```python
from build123d import *

# Parameters (mm, degrees)
SKETCH1_W           = 65
SKETCH1_H           = 46
SKETCH1_R           = 1.5
BOSS_EXTRUDE1_DEPTH = 5
SKETCH2_R           = 2
CUT_EXTRUDE1_DEPTH  = 10
SKETCH3_W           = 4
SKETCH3_H           = 46
CUT_EXTRUDE2_DEPTH  = 6
SKETCH4_W           = 6
SKETCH4_H           = 46
BOSS_EXTRUDE2_DEPTH = 5
FILLET1_R           = 10
FILLET2_R           = 1


with BuildPart() as part:
    # Sketch1 → Boss-Extrude1 (new body)
    with BuildSketch(Plane.XY):
        with Locations((7.5, 0)):
            Rectangle(SKETCH1_W, SKETCH1_H)
        with BuildLine():
            ThreePointArc((4.6, 0), (3.252691193, -3.252691193), (0, -4.6))
            ThreePointArc((0, -4.6), (-3.252691193, 3.252691193), (4.6, 0))
        make_face(mode=Mode.SUBTRACT)
        with Locations((30, -18.25)):
            Circle(SKETCH1_R, mode=Mode.SUBTRACT)
        with BuildLine():
            ThreePointArc((1.5, -10), (-1.060660172, -11.060660172), (0, -8.5))
            ThreePointArc((0, -8.5), (1.060660172, -8.939339828), (1.5, -10))
        make_face(mode=Mode.SUBTRACT)
        with BuildLine():
            ThreePointArc((39.5, 0), (23.282485579, -6.717514421), (30, 9.5))
            ThreePointArc((30, 9.5), (36.717514421, 6.717514421), (39.5, 0))
        make_face(mode=Mode.SUBTRACT)
        with Locations((0, 10)):
            Circle(SKETCH1_R, mode=Mode.SUBTRACT)
        with BuildLine():
            ThreePointArc((31.5, 18.25), (31.060660172, 17.189339828), (30, 16.75))
            ThreePointArc((30, 16.75), (28.939339828, 19.310660172), (31.5, 18.25))
        make_face(mode=Mode.SUBTRACT)
    extrude(amount=BOSS_EXTRUDE1_DEPTH)

    # Sketch2 → Cut-Extrude1 (cut)
    with BuildSketch(Plane.XY.offset(5)):
        with Locations((7, 19)):
            Circle(SKETCH2_R)
        with Locations((-5, -19)):
            Circle(SKETCH2_R)
        with Locations((-17, 19)):
            Circle(SKETCH2_R)
        with Locations((-5, 19)):
            Circle(SKETCH2_R)
        with Locations((7, -19)):
            Circle(SKETCH2_R)
        with Locations((-17, -19)):
            Circle(SKETCH2_R)
    extrude(amount=-CUT_EXTRUDE1_DEPTH, mode=Mode.SUBTRACT)

    # Sketch3 → Cut-Extrude2 (cut, through all)
    with BuildSketch(Plane.XY.offset(5)):
        with Locations((-23, 0)):
            Rectangle(SKETCH3_W, SKETCH3_H)
    extrude(amount=-CUT_EXTRUDE2_DEPTH, mode=Mode.SUBTRACT)

    # Sketch4 → Boss-Extrude2 (add)
    with BuildSketch(Plane.XY.offset(5)):
        with Locations((43, 0)):
            Rectangle(SKETCH4_W, SKETCH4_H)
    extrude(amount=-BOSS_EXTRUDE2_DEPTH)

    # Fillet1
    fillet1_edges = [part.edges().sort_by_distance(p)[0] for p in [
        (46, -23, 2.5),
        (46, 23, 2.5),
    ]]
    fillet(fillet1_edges, radius=FILLET1_R)

    # Fillet2
    fillet2_edges = [part.edges().sort_by_distance(p)[0] for p in [
        (-21, 23, 2.5),
        (-21, -23, 2.5),
    ]]
    fillet(fillet2_edges, radius=FILLET2_R)


solid = part.part
```
Geometry check sheet. Reference: the model listing, model coordinates, mm. Give positions to 0.01 mm unless a question says otherwise; leave off trailing zeros. Loops run counter-clockwise (first coordinate to the right, second up) from the corner with the lowest first, then second, coordinate; pieces in that order, holes last. Notation, with made-up numbers: M 80.5,12 L 131.5,12 A25 ccw 131.5,31 Z; hole C -19.75,83.5 d6. An arc over 180 degrees is marked long. Write item = value, one per line. Start each with the question number.
1. Section check B-B, the plane x = 27. Enter the section's corners in (y, z), plus the area to 3 significant figures.
2. Section check C-C, the plane y = 3. Enter the section's corners in (x, z), plus the area to 3 significant figures.
3. Thickness scan on probe 1 along X at (y, z) = (-1.5, 2.3); probe 2 along X at (y, z) = (4, 4.6); probe 3 along Y at (x, z) = (30, 1.7). Record the ranges inside material, lowest first.
4. Go/stop test with a flat-tipped pin: P1, Ø15, axis at x = 30, y = 0, coming from the -Z side. Record where the tip stops, or that it passes through.
5. Draft check along X on faces 1 (the face through (-17, -17, 3)), 2 (the face through (-21, 0, 3)), 3 (the face through (8, -23, 3)), 4 (the face through (-5, 21, 3)). Enter one of: +X half, -X half, draft (parallel to the pull), parting line (faces both ways), or undercut.
6. Section check D-D, the plane y = 19. Enter the section's corners in (x, z), plus the area to 3 significant figures.
7. Section check A-A, the plane z = 1.8. Give the number of separate pieces and of enclosed holes in the cut face, plus the area to 3 significant figures.
Values follow:
q1.outline = M -23,0 L -9.01,0 L -9.01,5 L -23,5 Z; M 9.01,0 L 23,0 L 23,5 L 9.01,5 Z
q1.area = 140 mm^2
q2.outline = M -21,0 L -3.49,0 L -3.49,5 L -21,5 Z; M 3.49,0 L 20.99,0 L 20.99,5 L 3.49,5 Z; M 39.01,0 L 46,0 L 46,5 L 39.01,5 Z
q2.area = 210 mm^2
q3.probe_1 = -21 to -4.35, 4.35 to 20.62, 39.38 to 46
q3.probe_2 = -21 to -2.27, 2.27 to 21.38, 38.62 to 46
q3.probe_3 = -23 to -19.75, -16.75 to -9.5, 9.5 to 16.75, 19.75 to 23
q4.P1 = through
q5.face_1 = undercut
q5.face_2 = -X half
q5.face_3 = draft
q5.face_4 = undercut
q6.outline = M -21,0 L -19,0 L -19,5 L -21,5 Z; M -15,0 L -7,0 L -7,5 L -15,5 Z; M -3,0 L 5,0 L 5,5 L -3,5 Z; M 9,0 L 28.7,0 L 28.7,5 L 9,5 Z; M 31.3,0 L 44,0 L 44,5 L 31.3,5 Z
q6.area = 252 mm^2
q7.separate_pieces = 1
q7.enclosed_holes = 12
q7.area = 2,580 mm^2
